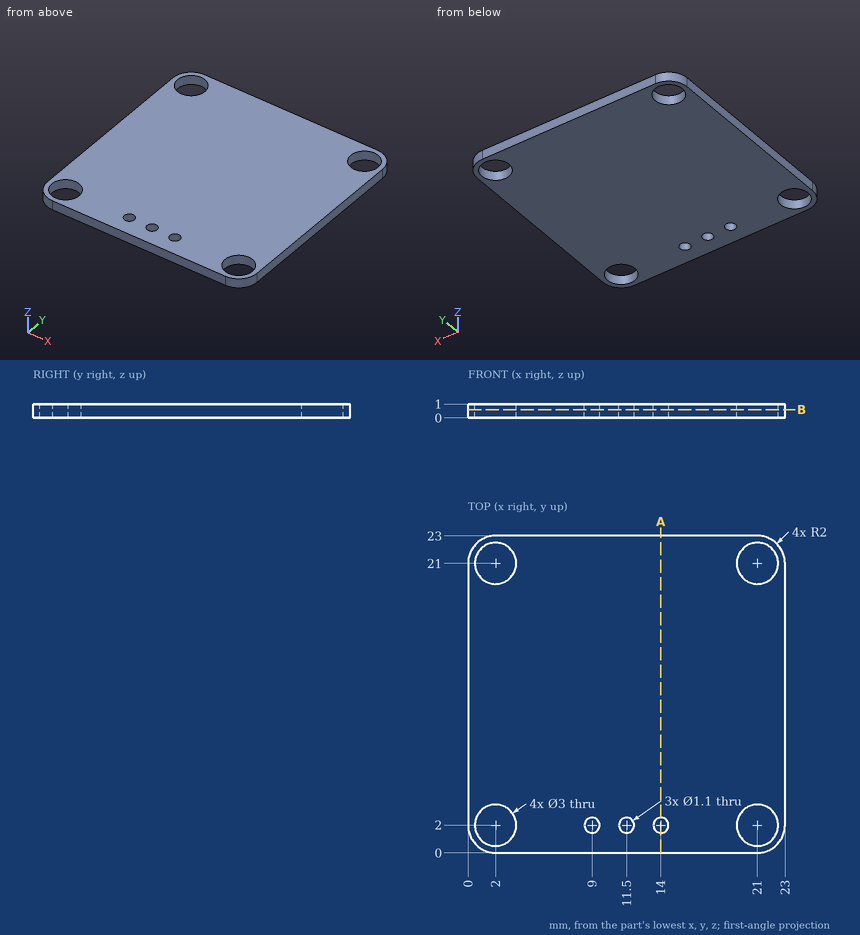
Check sheet for the drawn part. Datum: minimum x, y, z corner. Units: mm. Coordinates: 2 decimals unless noted, no trailing zeros. Order: outer loops, then holes, each group sorted by start corner. A loop starts at its lowest first (then second) coordinate and runs counter-clockwise, first axis right, second up. Notation, with made-up numbers: M 66.25,69.5 L 76.25,69.5 A21 cw 76.25,103.5 Z; hole C 14,42.25 d1. An arc over 180 degrees is marked long. One line per item, written item: value. Start each with the question number.
Item 1: Scan lines: probe 1 along X at (y, z) = (2, 0.55); probe 2 along Y at (x, z) = (21, 0.35). Record each from-to range of solid material in increasing order.
Item 2: Gauge pin test, flat end, axial feed: pin 1 (6 mm diameter, centred on x = 10.5, y = 12.5, fed in from -Z). Record the tip position at first contact, or that the pin passes through.
Item 3: Sectioned sample at B-B (z = 0.6). Enter the section's corners in (x, y).
Item 4: Sectioned sample at A-A (x = 14). Enter the section's corners in (y, z), then the cut area to 3 significant figures.
Conclusion:
1. probe 1: x = 0 to 0.5, 3.5 to 8.45, 9.55 to 10.95, 12.05 to 13.45, 14.55 to 19.5, 22.5 to 23
1. probe 2: y = 0 to 0.5, 3.5 to 19.5, 22.5 to 23
2. pin 1: stops at z = 0
3. outline: M 0,2 A2 ccw 2,0 L 21,0 A2 ccw 23,2 L 23,21 A2 ccw 21,23 L 2,23 A2 ccw 0,21 Z; hole C 2,2 d3; hole C 2,21 d3; hole C 9,2 d1.1; hole C 11.5,2 d1.1; hole C 14,2 d1.1; hole C 21,2 d3; hole C 21,21 d3
4. outline: M 0,0 L 1.45,0 L 1.45,1 L 0,1 Z; M 2.55,0 L 23,0 L 23,1 L 2.55,1 Z
4. area: 21.9 mm^2
